from build123d import *

# Parameters (mm, degrees)
SKETCH1_W          = 6
SKETCH1_H          = 12.5
SKETCH1_W_2        = 8
SKETCH7_W          = 10
SKETCH7_H          = 12.5
CUT_EXTRUDE1_REACH = 95.493
SKETCH8_R          = 4
CUT_EXTRUDE2_REACH = 87.277
CUT_EXTRUDE3_DEPTH = 20


with BuildPart() as part:
    # Sketch1 → Revolve1 (revolve)
    with BuildSketch(Plane(origin=(0, 0, 0), x_dir=(1, 0, 0), z_dir=(0, 1, 0)), mode=Mode.PRIVATE) as revolve1_sk:
        Polygon((5, 12.5), (0, 20), (0, 40), (5, 40), (10.459553514, 25), (19.540446486, 25), (25, 40), (30, 40), (30, 25), (36, 25), (36, 12.5), align=None)
        with Locations((47, 18.75)):
            Rectangle(SKETCH1_W, SKETCH1_H)
        with Locations((40, 18.75)):
            Rectangle(SKETCH1_W_2, SKETCH1_H)
    revolve(revolve1_sk.sketch.rotate(Axis((-23.221484356, 0, 0), (1, 0, 0)), 180), axis=Axis((-23.221484356, 0, 0), (1, 0, 0)))

    # Sketch7 → Revolve-Thin2 (revolve)
    with BuildSketch(Plane(origin=(0, 0, 0), x_dir=(1, 0, 0), z_dir=(0, 1, 0))):
        with Locations((31, 18.75)):
            Rectangle(SKETCH7_W, SKETCH7_H)
    revolve(axis=Axis((40, 0, -25), (0, 0, 1)))

    # Sketch8 → Cut-Extrude1 (cut, up to next)
    with BuildSketch(Plane(origin=(0, 0, -25), x_dir=(-1, 0, 0), z_dir=(0, 0, -1)), mode=Mode.PRIVATE) as cut_extrude1_sk1:
        with Locations((-40, 0)):
            Circle(SKETCH8_R)
    cut_extrude1_tool1 = extrude(cut_extrude1_sk1.sketch, amount=-CUT_EXTRUDE1_REACH, mode=Mode.PRIVATE) & part.part
    add(cut_extrude1_tool1.solids().sort_by_distance((40, 0, -25))[0], mode=Mode.SUBTRACT)

    # Sketch9 → Cut-Extrude2 (cut, up to next)
    with BuildSketch(Plane.XY.offset(-12.5), mode=Mode.PRIVATE) as cut_extrude2_sk1:
        with BuildLine():
            Line((50, 9.797958971), (50, -9.797958971))
            ThreePointArc((50, -9.797958971), (54, 0), (50, 9.797958971))
        make_face()
    cut_extrude2_tool1 = extrude(cut_extrude2_sk1.sketch, amount=-CUT_EXTRUDE2_REACH, mode=Mode.PRIVATE) & part.part
    add(cut_extrude2_tool1.solids().sort_by_distance((51.621368, 0, -12.5))[0], mode=Mode.SUBTRACT)

    # Sketch12 → Cut-Extrude3 (cut)
    with BuildSketch(Plane(origin=(50, 0, 0), x_dir=(0, 0, -1), z_dir=(1, 0, 0))):
        with BuildLine():
            Line((25, 9.797958971), (25, 14))
            Line((25, 14), (20.712315177, 14))
            ThreePointArc((20.712315177, 14), (21.956910341, 11.953831531), (23, 9.797958971))
            Line((23, 9.797958971), (25, 9.797958971))
        make_face()
        with BuildLine():
            Line((25, 0), (25, 9.797958971))
            Line((25, 9.797958971), (23, 9.797958971))
            ThreePointArc((23, 9.797958971), (24.494897428, 5), (25, 0))
        make_face()
        with BuildLine():
            ThreePointArc((23, -9.797958971), (21.956910341, -11.953831531), (20.712315177, -14))
            Line((20.712315177, -14), (25, -14))
            Line((25, -14), (25, -9.797958971))
            Line((25, -9.797958971), (23, -9.797958971))
        make_face()
        with BuildLine():
            Line((25, -9.797958971), (25, 0))
            ThreePointArc((25, 0), (24.494897428, -5), (23, -9.797958971))
            Line((23, -9.797958971), (25, -9.797958971))
        make_face()
    extrude(amount=-CUT_EXTRUDE3_DEPTH, mode=Mode.SUBTRACT)


solid = part.part
Input: part model. Units: mm. Frame: model coordinates. A direction names the side the tool comes from. Coordinates: 2 decimals unless noted, no trailing zeros. Loops run counter-clockwise (first coordinate to the right, second up) from the corner with the lowest first, then second, coordinate; pieces in that order, holes last.
(1) Section B-B on x = 40. Return the cut outline in (y, z).
(2) Pull-direction query (Y, two-part tool) for faces 5 (the face through (2.54, -1.76, -39.96)), 6 (the face through (27.815, -3.755, 11.923)), 7 (the face through (0, -18.3, 9.4)); classes: released by +Y, released by -Y, zero draft, split by the parting line, or undercut.
(3) Section A-A on z = 0. Return the cut outline in (x, y).
(4) Set-up query: faces 1 (the face through (30, -18.34, 17.22)), 2 (the face through (19.88, -7.79, 24.74)), 3 (the face through (43.2, -2.4, -18.5)), 4 (the face through (50, -5.9, 11.5)). Return all of +Z, -Z, +X, -X, +Y, -Y with unobstructed straight access to the full face (end or side cutting, diameter ignored); none if empty.
(5) First-contact query: pin 1 Ø13 at (x, y) = (40, 0) entering from -Z; pin 2 Ø4 at (x, z) = (34.5, 15.5) entering from -Y; pin 3 Ø15 at (y, z) = (0, 0) entering from -X; pin 4 Ø5 at (y, z) = (-27.5, 21.5) entering from -X. Flat tips, straight axial feed; report the tip coordinate or a pass-through.
(6) Section C-C on y = 1. Count the separate pieces of the cut face and the enclosed holes in it, then the cut area to 3 significant figures.
(7) Material intervals for probe 1 along Y at (x, z) = (18, 0); probe 2 along Y at (x, z) = (28.5, 0); probe 3 along X at (y, z) = (0, -21), sorted ascending.
Data:
1. outline: (-4, -24.68) - (-4, -11.84) arc R12.5 cw (long way) to (4, -11.84) - (4, -24.68) arc R25 ccw (long way) to start
2. face 5: split by the parting line
2. face 6: undercut
2. face 7: zero draft
3. outline: (0, -40) - (5, -40) - (10.46, -25) - (19.54, -25) - (25, -40) - (30, -40) - (30, -25) - (50, -25) - (50, -12.5) - (5, -12.5) - (0, -20) - close; (0, 20) - (5, 12.5) - (50, 12.5) - (50, 25) - (30, 25) - (30, 40) - (25, 40) - (19.54, 25) - (10.46, 25) - (5, 40) - (0, 40) - close
4. face 1: +X
4. face 2: none
4. face 3: -Z
4. face 4: +Z, -Z, +X, +Y, -Y
5. pin 1: stops at z = -25
5. pin 2: stops at y = -21.04
5. pin 3: passes through
5. pin 4: stops at x = 0
6. separate pieces: 3
6. enclosed holes: 0
6. area: 1,580 mm2
7. probe 1: y = -25 to -12.5, 12.5 to 25
7. probe 2: y = -40 to -12.5, 12.5 to 40
7. probe 3: x = 0 to 36, 44 to 50
